from build123d import *

# Parameters (mm, degrees)
SKETCH_W        = 100
SKETCH_H        = 70
PAD_DEPTH       = 10
SKETCH001_W     = 100
SKETCH001_H     = 10
PAD001_DEPTH    = 20
SKETCH002_W     = 93.4
SKETCH002_H     = 5
POCKET_DEPTH    = 15
SKETCH003_W     = 3
SKETCH003_H     = 3
PAD002_DEPTH    = 10
SKETCH004_R     = 1.7
POCKET001_DEPTH = 15
SKETCH005_R     = 3
POCKET002_DEPTH = 3.2
FILLET_R        = 5
FILLET001_R     = 1
FILLET002_R     = 1


with BuildPart() as part:
    # Sketch → Pad (new body)
    with BuildSketch(Plane.XY):
        with Locations((50, 35)):
            Rectangle(SKETCH_W, SKETCH_H)
    extrude(amount=PAD_DEPTH)

    # Sketch001 → Pad001 (new body)
    with BuildSketch(Plane(origin=(0, 0, 0), x_dir=(1, 0, 0), z_dir=(0, 0, -1))):
        with Locations((50, -5)):
            Rectangle(SKETCH001_W, SKETCH001_H)
    extrude(amount=PAD001_DEPTH)

    # Sketch002 → Pocket (cut)
    with BuildSketch(Plane(origin=(0, 70, 0), x_dir=(-1, 0, 0), z_dir=(0, 1, 0))):
        with Locations((-50, 7.5)):
            Rectangle(SKETCH002_W, SKETCH002_H)
    extrude(amount=-POCKET_DEPTH, mode=Mode.SUBTRACT)

    # Sketch003 → Pad002 (new body)
    with BuildSketch(Plane(origin=(0, 55, 0), x_dir=(-1, 0, 0), z_dir=(0, 1, 0))):
        with Locations((-6.5, 8.2)):
            Rectangle(SKETCH003_W, SKETCH003_H)
        with Locations((-93.5, 8.2)):
            Rectangle(SKETCH003_W, SKETCH003_H)
    extrude(amount=PAD002_DEPTH)

    # Sketch004 → Pocket001 (cut)
    with BuildSketch(Plane(origin=(0, 10, 0), x_dir=(-1, 0, 0), z_dir=(0, 1, 0))):
        with Locations((-20, -10)):
            Circle(SKETCH004_R)
        with Locations((-80, -10)):
            Circle(SKETCH004_R)
    extrude(amount=-POCKET001_DEPTH, mode=Mode.SUBTRACT)

    # Sketch005 → Pocket002 (cut)
    with BuildSketch(Plane(origin=(0, 10, 0), x_dir=(-1, 0, 0), z_dir=(0, 1, 0))):
        with Locations((-20, -10)):
            Circle(SKETCH005_R)
        with Locations((-80, -10)):
            Circle(SKETCH005_R)
    extrude(amount=-POCKET002_DEPTH, mode=Mode.SUBTRACT)

    # Fillet
    fillet_edges = [part.edges().sort_by_distance(p)[0] for p in [
        (50, 10, 0),
    ]]
    fillet(fillet_edges, radius=FILLET_R)

    # Fillet001
    fillet001_edges = [part.edges().sort_by_distance(p)[0] for p in [
        (100, 70, 5),
        (50, 70, 0),
        (100, 42.5, 0),
        (100, 35, 10),
        (100, 11.464466, -1.464466),
        (100, 10, -12.5),
        (50, 10, -20),
        (100, 5, -20),
        (0, 5, -20),
        (0, 10, -12.5),
        (0, 11.464466, -1.464466),
        (0, 42.5, 0),
        (0, 70, 5),
        (0, 35, 10),
        (1.65, 70, 10),
        (98.35, 70, 10),
        (92, 65, 8.2),
        (93.5, 65, 6.7),
        (95, 65, 8.2),
        (93.5, 65, 9.7),
        (5, 65, 8.2),
        (6.5, 65, 6.7),
        (8, 65, 8.2),
        (6.5, 65, 9.7),
        (3.3, 70, 7.5),
        (50, 70, 5),
        (96.7, 70, 7.5),
    ]]
    fillet(fillet001_edges, radius=FILLET001_R)

    # Fillet002
    fillet002_edges = [part.edges().sort_by_distance(p)[0] for p in [
        (95, 55, 8.2),
        (92, 55, 8.2),
        (8, 55, 8.2),
        (5, 55, 8.2),
    ]]
    fillet(fillet002_edges, radius=FILLET002_R)


solid = part.part
Could you check a few things on this model? Use its own coordinates, in mm. A direction names the side the tool comes from. Give positions to 0.01 mm unless a question says otherwise; leave off trailing zeros. Loops run counter-clockwise (first coordinate to the right, second up) from the corner with the lowest first, then second, coordinate; pieces in that order, holes last. Notation, with made-up numbers: (75.25, -11.5) -> (121.25, -11.5) arc R17 cw to (121.25, 5.5) -> close; hole circle Ø6 at (-27.5, 55). An arc over 180 degrees is marked (long way). Return JSON: item names as keys, results as strings.
Item 1: I'm going to push flat-ended pins straight in: pin 1 (4 mm diameter, centred on x = 92.5, y = 61.5, fed in from +Z); pin 2 (4 mm diameter, centred on x = 71.5, z = 8.5, fed in from +Y); pin 3 (8 mm diameter, centred on x = 51, z = -7.5, fed in from +Y); pin 4 (1 mm diameter, centred on x = 74.5, z = -11.5, fed in from -Y). Where does each tip first touch, or does it pass through?
Geometry results:
{"pin 1": "stops at z = 9.7", "pin 2": "stops at y = 55", "pin 3": "stops at y = 10.23", "pin 4": "stops at y = 0"}
Item 2: If we section it at B-B on x = 80: List the corners of the cut face in (y, z) for me, plus the area to 3 significant figures.
Geometry results:
{"outline": "(0, -20) -> (9, -20) arc R1 ccw to (10, -19) -> (10, -13) -> (6.8, -13) -> (6.8, -11.7) -> (0, -11.7) -> close; (0, -8.3) -> (6.8, -8.3) -> (6.8, -7) -> (10, -7) -> (10, -5) arc R5 cw to (15, 0) -> (69, 0) arc R1 ccw to (70, 1) -> (70, 4) arc R1 ccw to (69, 5) -> (55, 5) -> (55, 10) -> (0, 10) -> close", "area": "787 mm²"}
Item 3: If we section it at D-D on y = 17: List the corners of the cut face in (x, z) for me.
Geometry results:
{"outline": "(0, 1) arc R1 ccw to (1, 0) -> (99, 0) arc R1 ccw to (100, 1) -> (100, 9) arc R1 ccw to (99, 10) -> (1, 10) arc R1 ccw to (0, 9) -> close"}
Item 4: Which directions (+Z, -Z, +X, -X, +Y, -Y) give clear straight access to the entire face, cutting with the end or side of a thin tool? Please do faces 1 (the cylindrical face through (83, 8, -10)), 2 (the flat face through (3.3, 62, 7)), 3 (the flat face through (49, 10, -12)), 4 (the flat face through (49, 4, -20)).
Geometry results:
{"face 1": "+Y", "face 2": "+Z, +Y", "face 3": "-Z, +X, -X, +Y", "face 4": "-Z, +X, -X, +Y, -Y"}
Item 5: We'd pull the mould along Z, two halves only. Please class faces 5 (the flat face through (49, 42, 0)), 6 (the flat face through (100, 27.3, 1.4)), 7 (the flat face through (80, 6.8, -12)): +Z half, -Z half, draft (parallel to the pull), parting line (faces both ways), or undercut.
Geometry results:
{"face 5": "-Z half", "face 6": "draft", "face 7": "undercut"}
Item 6: I need wall thicknesses on L1, parallel to Z at x = 80, y = 5.5; L2, parallel to Z at x = 20, y = 8.05; L3, parallel to Z at x = 25, y = 19. Which ranges of each line are inside material? Lowest first, please. Write a range as from..to.
Geometry results:
{"L1": "z = -20..-11.7, -8.3..10", "L2": "z = -20..-13, -7..10", "L3": "z = 0..10"}
Item 7: If we section it at A-A on y = 60.5: List the corners of the cut face in (x, z) for me, plus the area to 3 significant figures.
Geometry results:
{"outline": "(0, 1) arc R1 ccw to (1, 0) -> (99, 0) arc R1 ccw to (100, 1) -> (100, 9) arc R1 ccw to (99, 10) -> (96.7, 10) -> (96.7, 5) -> (3.3, 5) -> (3.3, 10) -> (1, 10) arc R1 ccw to (0, 9) -> close; (5, 6.7) -> (8, 6.7) -> (8, 9.7) -> (5, 9.7) -> close; (92, 6.7) -> (95, 6.7) -> (95, 9.7) -> (92, 9.7) -> close", "area": "550 mm²"}
Item 8: If we section it at C-C on x = 66.5: List the corners of the cut face in (y, z) for me, plus the area to 3 significant figures.
Geometry results:
{"outline": "(0, -20) -> (9, -20) arc R1 ccw to (10, -19) -> (10, -5) arc R5 cw to (15, 0) -> (69, 0) arc R1 ccw to (70, 1) -> (70, 4) arc R1 ccw to (69, 5) -> (55, 5) -> (55, 10) -> (0, 10) -> close", "area": "830 mm²"}
